```python
from build123d import *

# Parameters (mm, degrees)
SKETCH_1_W          = 3
SKETCH_1_H          = 90
EXTRUDE_1_DEPTH     = 80
SKETCH_2_R          = 2.6
CUT_EXTRUDE_1_DEPTH = 118.276484819
SKETCH_3_W          = 49.268401117
SKETCH_3_H          = 61
CUT_EXTRUDE_2_DEPTH = 118.276484819
SKETCH_4_R          = 2.55
CUT_EXTRUDE_3_DEPTH = 121.608375453
CUT_EXTRUDE_4_DEPTH = 121.608375453
FILLET_2_R          = 5
SKETCH_6_W          = 50
SKETCH_6_H          = 43.1
CUT_EXTRUDE_6_DEPTH = 121.608375453
FILLET_3_R          = 5


with BuildPart() as part:
    # 草图1 → 凸台-拉伸1 (new body)
    with BuildSketch(Plane.XY):
        Polygon((-1.18201613, 42.576507787), (-31.965089897, 81.977045467), (-29.601057636, 83.824029893), (1.18201613, 44.423492213), align=None)
        Rectangle(SKETCH_1_W, SKETCH_1_H)
    extrude(amount=EXTRUDE_1_DEPTH)

    # 草图2 → 切除-拉伸1 (cut, through all)
    with BuildSketch(Plane(origin=(22.285948177, 17.411690984, 0), x_dir=(0.6156614753256597, -0.788010753606721, 0), z_dir=(0.788010753606721, 0.6156614753256597, 0))):
        with Locations(Location((-80.278467782, -4, 0), (0, 0, 180))):
            Circle(SKETCH_2_R)
        with Locations(Location((-80.278467782, -76, 0), (0, 0, 180))):
            Circle(SKETCH_2_R)
        with Locations(Location((-40.278467782, -4, 0), (0, 0, 180))):
            Circle(SKETCH_2_R)
        with Locations(Location((-40.278467782, -76, 0), (0, 0, 180))):
            Circle(SKETCH_2_R)
    extrude(amount=-CUT_EXTRUDE_1_DEPTH, mode=Mode.SUBTRACT)

    # 草图3 → 切除-拉伸2 (cut, through all)
    with BuildSketch(Plane(origin=(22.285948177, 17.411690984, 0), x_dir=(0.6156614753256597, -0.788010753606721, 0), z_dir=(0.788010753606721, 0.6156614753256597, 0))):
        with Locations((-59.644267224, -40)):
            Rectangle(SKETCH_3_W, SKETCH_3_H)
    extrude(amount=-CUT_EXTRUDE_2_DEPTH, mode=Mode.SUBTRACT)

    # 草图4 → 切除-拉伸3 (cut, through all)
    with BuildSketch(Plane(origin=(1.5, 0, 0), x_dir=(0, 0, -1), z_dir=(1, 0, 0))):
        with Locations(Location((-65, -28.3, 0), (0, 0, 90))):
            Circle(SKETCH_4_R)
        with Locations(Location((-65, -41, 0), (0, 0, 90))):
            Circle(SKETCH_4_R)
        with Locations(Location((-52.3, -28.3, 0), (0, 0, 90))):
            Circle(SKETCH_4_R)
        with Locations(Location((-52.3, -41, 0), (0, 0, 90))):
            Circle(SKETCH_4_R)
        with Locations(Location((-39.6, -28.3, 0), (0, 0, 90))):
            Circle(SKETCH_4_R)
        with Locations(Location((-39.6, -41, 0), (0, 0, 90))):
            Circle(SKETCH_4_R)
        with Locations(Location((-26.9, -28.3, 0), (0, 0, 90))):
            Circle(SKETCH_4_R)
        with Locations(Location((-26.9, -41, 0), (0, 0, 90))):
            Circle(SKETCH_4_R)
    extrude(amount=-CUT_EXTRUDE_3_DEPTH, mode=Mode.SUBTRACT)

    # 草图5 → 切除-拉伸4 (cut, through all)
    with BuildSketch(Plane(origin=(1.5, 0, 0), x_dir=(0, 0, -1), z_dir=(1, 0, 0))):
        with BuildLine():
            Line((-80, 6.141923624), (-80, -45))
            Line((-80, -45), (-71.424177932, -45))
            ThreePointArc((-71.424177932, -45), (-70.206204317, -18.505774381), (-80, 6.141923624))
        make_face()
        with BuildLine():
            Line((0, -45), (-8.575822068, -45))
            ThreePointArc((-8.575822068, -45), (-9.793795683, -18.505774381), (0, 6.141923624))
            Line((0, 6.141923624), (0, -45))
        make_face()
    extrude(amount=-CUT_EXTRUDE_4_DEPTH, mode=Mode.SUBTRACT)

    # 圆角2
    # the kernel refuses this fillet: 5 mm, written as the material it adds along each edge
    with BuildSketch(Plane(origin=(-1.5, 42.98350858, 80), x_dir=(-0.61566147532566, 0.7880107536067206, 0), z_dir=(0, 0, -1))) as fillet_2_piece_1_section:
        with BuildLine():
            CenterArc((FILLET_2_R * 0.34432761329, -FILLET_2_R), FILLET_2_R, 90, 38)
            Line((-FILLET_2_R * 0.271333862036, -FILLET_2_R * 0.211989246393), (0, 0))
            Line((0, 0), (FILLET_2_R * 0.34432761329, 0))
        make_face()
    fillet_2_piece_1 = extrude(amount=84.304095166, mode=Mode.PRIVATE)
    fillet_2_piece_1 = split(fillet_2_piece_1, bisect_by=Plane(origin=(-1.5, 42.98350858, 70.5), z_dir=(0, 0, 1)), keep=Keep.TOP, mode=Mode.PRIVATE)
    add(fillet_2_piece_1)
    with BuildSketch(Plane(origin=(-1.5, 42.98350858, 84.304095166), x_dir=(-0.61566147532566, 0.7880107536067206, 0), z_dir=(0, 0, -1))) as fillet_2_piece_2_section:
        with BuildLine():
            CenterArc((FILLET_2_R * 0.34432761329, -FILLET_2_R), FILLET_2_R, 90, 38)
            Line((-FILLET_2_R * 0.271333862036, -FILLET_2_R * 0.211989246393), (0, 0))
            Line((0, 0), (FILLET_2_R * 0.34432761329, 0))
        make_face()
    fillet_2_piece_2 = extrude(amount=84.304095166, mode=Mode.PRIVATE)
    fillet_2_piece_2 = split(fillet_2_piece_2, bisect_by=Plane(origin=(-1.632433378, 43.153015574, 84.304095166), z_dir=(0.6156614753256597, -0.7880107536067209, 0)), keep=Keep.TOP, mode=Mode.PRIVATE)
    fillet_2_piece_2 = split(fillet_2_piece_2, bisect_by=Plane(origin=(-1.5, 42.98350858, 70.5), z_dir=(0, 0, -1)), keep=Keep.TOP, mode=Mode.PRIVATE)
    add(fillet_2_piece_2)
    with BuildSketch(Plane(origin=(-1.5, 42.98350858, 84.304095166), x_dir=(-0.61566147532566, 0.7880107536067206, 0), z_dir=(0, 0, -1))) as fillet_2_piece_3_section:
        with BuildLine():
            CenterArc((FILLET_2_R * 0.34432761329, -FILLET_2_R), FILLET_2_R, 90, 38)
            Line((-FILLET_2_R * 0.271333862036, -FILLET_2_R * 0.211989246393), (0, 0))
            Line((0, 0), (FILLET_2_R * 0.34432761329, 0))
        make_face()
    fillet_2_piece_3 = extrude(amount=84.304095166, mode=Mode.PRIVATE)
    fillet_2_piece_3 = split(fillet_2_piece_3, bisect_by=Plane(origin=(-1.5, 42.98350858, 9.5), z_dir=(0, 0, -1)), keep=Keep.TOP, mode=Mode.PRIVATE)
    add(fillet_2_piece_3)
    # the kernel refuses this fillet: 5 mm, written as the material it takes off along each edge
    with BuildSketch(Plane(origin=(1.5, 45, -6.658439614), x_dir=(0, -1, 0), z_dir=(0, 0, 1))) as fillet_2_2_piece_1:
        with BuildLine():
            CenterArc((2.663375846, -5), FILLET_2_R, 90, 32.186384057)
            Line((0, -0.768401117), (0, 0))
            Line((0, 0), (2.663375846, 0))
        make_face()
    extrude(amount=93.316879228, mode=Mode.SUBTRACT)

    # 草图6 → 切除-拉伸6 (cut, through all)
    with BuildSketch(Plane(origin=(1.5, 0, 0), x_dir=(0, 0, -1), z_dir=(1, 0, 0))):
        with Locations((-39.698542008, 15.9)):
            Rectangle(SKETCH_6_W, SKETCH_6_H)
    extrude(amount=-CUT_EXTRUDE_6_DEPTH, mode=Mode.SUBTRACT)

    # 圆角3
    # the kernel refuses this fillet: 5 mm, written as the material it adds along each edge
    with BuildSketch(Plane(origin=(1.5, -5.65, 14.698542008), x_dir=(0, 1, 0), z_dir=(-1, 0, 0)), Plane(origin=(1.5, -5.65, 64.698542008), x_dir=(0, 0, -1), z_dir=(-1, 0, 0)), Plane(origin=(1.5, 37.45, 64.698542008), x_dir=(0, -1, 0), z_dir=(-1, 0, 0))) as fillet_3_piece_1:
        with BuildLine():
            CenterArc((FILLET_3_R, -FILLET_3_R), FILLET_3_R, 90, 90)
            Line((0, -FILLET_3_R), (0, 0))
            Line((0, 0), (FILLET_3_R, 0))
        make_face()
    extrude(amount=3)
    with BuildSketch(Plane(origin=(1.5, 37.45, 14.698542008), x_dir=(0, -1, 0), z_dir=(-1, 0, 0))) as fillet_3_piece_2:
        with BuildLine():
            CenterArc((FILLET_3_R, FILLET_3_R), FILLET_3_R, 180, 90)
            Line((0, FILLET_3_R), (0, 0))
            Line((0, 0), (FILLET_3_R, 0))
        make_face()
    extrude(amount=3)
    # the kernel refuses this fillet: 5 mm, written as the material it takes off along each edge
    with BuildSketch(Plane(origin=(-41.815224317, 74.281277026, 0), x_dir=(0.6156614753256596, -0.7880107536067208, 0), z_dir=(0.7880107536067208, 0.6156614753256597, 0)), Plane(origin=(-19.750923216, 91.519798335, 9.5), x_dir=(0.6156614753256597, -0.7880107536067208, 1.0658141036401496e-15), z_dir=(-0.7880107536067209, -0.6156614753256597, 0))) as fillet_3_2_piece_1:
        with BuildLine():
            CenterArc((FILLET_3_R, -FILLET_3_R), FILLET_3_R, 90, 90)
            Line((0, -FILLET_3_R), (0, 0))
            Line((0, 0), (FILLET_3_R, 0))
        make_face()
    extrude(amount=28, mode=Mode.SUBTRACT)
    with BuildSketch(Plane(origin=(-41.815224317, 74.281277026, 80), x_dir=(0.6156614753256597, -0.7880107536067208, 0), z_dir=(0.7880107536067208, 0.6156614753256597, 0)), Plane(origin=(-19.750923216, 91.519798335, 70.5), x_dir=(0.6156614753256597, -0.7880107536067208, 0), z_dir=(-0.7880107536067209, -0.6156614753256597, 0))) as fillet_3_2_piece_2:
        with BuildLine():
            CenterArc((FILLET_3_R, FILLET_3_R), FILLET_3_R, 180, 90)
            Line((0, FILLET_3_R), (0, 0))
            Line((0, 0), (FILLET_3_R, 0))
        make_face()
    extrude(amount=28, mode=Mode.SUBTRACT)
    with BuildSketch(Plane(origin=(5.221396316, 6.141923624, 0), x_dir=(0, 1, 0), z_dir=(-1, 0, 0))) as fillet_3_2_piece_3:
        with BuildLine():
            CenterArc((1.488558526, -5), FILLET_3_R, 90, 32.518664638)
            ThreePointArc((-1.199313086, -0.783918147), (-0.597427923, -0.395368629), (0, 0))
            Line((0, 0), (1.488558526, 0))
        make_face()
    extrude(amount=10.442792632, mode=Mode.SUBTRACT)
    with BuildSketch(Plane(origin=(5.221396316, 6.141923624, 80), x_dir=(0, 1, 0), z_dir=(-1, 0, 0))) as fillet_3_2_piece_4:
        with BuildLine():
            CenterArc((1.488558526, 5), FILLET_3_R, 237.481335362, 32.518664638)
            ThreePointArc((-1.199313086, 0.783918147), (-0.597427923, 0.395368629), (0, 0))
            Line((0, 0), (1.488558526, 0))
        make_face()
    extrude(amount=10.442792632, mode=Mode.SUBTRACT)
    with BuildSketch(Plane(origin=(16.943632487, -45, 71.424177932), x_dir=(0, 0, -1), z_dir=(-1, 0, 0))) as fillet_3_2_piece_5:
        with BuildLine():
            CenterArc((6.177452995, -5), FILLET_3_R, 90, 99.373749783)
            ThreePointArc((1.244218563, -5.814369722), (0.69074329, -2.892497851), (0, 0))
            Line((0, 0), (6.177452995, 0))
        make_face()
    extrude(amount=33.887264974, mode=Mode.SUBTRACT)
    with BuildSketch(Plane(origin=(16.943632487, -45, 8.575822068), x_dir=(0, 0.9778615645016191, 0.20925286299223153), z_dir=(-1, 0, 0))) as fillet_3_2_piece_6:
        with BuildLine():
            CenterArc((6.181957548, -4.994429535), FILLET_3_R, 92.704821928, 99.373749783)
            Line((1.292649725, -6.04069385), (0, 0))
            ThreePointArc((0, 0), (2.973002485, -0.070187858), (5.946004969, 0))
        make_face()
    extrude(amount=33.887264974, mode=Mode.SUBTRACT)


solid = part.part
```
Build history of the part. All positions in model axes, mm. A direction names the side the tool comes from. Coordinates: 2 decimals unless noted, no trailing zeros. Write each loop counter-clockwise with the first axis right and the second up, starting at its lowest first coordinate (ties: lowest second). Pieces come first, ordered by that corner, then holes.
1. Band-saw the part on D-D, the plane z = 18. Give the cut face in (x, y), and give its area (3 significant figures).
Answer block:
outline: (-1.82, 43.01) arc R5 cw to (-1.5, 41.26) - (-1.5, 37.15) - (1.5, 37.15) - (1.5, 42.34) arc R5 ccw to (0.73, 45) - close; (-1.5, -45) - (1.5, -45) - (1.5, -5.35) - (-1.5, -5.35) - close
area: 140 mm2
2. 3-axis set-ups, long thin cutter, end or side, ignore diameter. For faces 5 (the flat face through (-0.52, 44.02, 39.57)), 6 (the cylindrical face through (-29.82, 81.63, 1.34)), 7 (the cylindrical face through (0.02, 35.95, 63.27)): which of +Z, -Z, +X, -X, +Y, -Y reach the whole face in a straight line?
Answer block:
face 5: -X, +Y
face 6: -Z, -X, +Y
face 7: +X, -X
3. Band-saw the part on A-A, the plane y = 22. Give the cut face in (x, z).
Answer block:
outline: (-1.5, 0) - (1.5, 0) - (1.5, 14.7) - (-1.5, 14.7) - close; (-1.5, 64.7) - (1.5, 64.7) - (1.5, 80) - (-1.5, 80) - close
4. Drop flat-ended pins along their axis: pin 1 (5 mm diameter, centred on x = -22, z = 66.5, fed in from -Y); pin 2 (2 mm diameter, centred on y = -24.5, z = 64.5, fed in from -X); pin 3 (0.9 mm diameter, centred on x = -0.5, z = 47, fed in from +Y). Give the stop position or say it passes through.
Answer block:
pin 1: passes through
pin 2: stops at x = -1.5
pin 3: stops at y = 44.39
5. Band-saw the part on B-B, the plane z = 52.3. Give the cut face in (x, y), and give its area (3 significant figures).
Answer block:
outline: (-1.82, 43.01) arc R5 cw to (-1.5, 41.26) - (-1.5, 37.45) - (1.5, 37.45) - (1.5, 42.34) arc R5 ccw to (0.73, 45) - close; (-1.5, -45) - (1.5, -45) - (1.5, -43.55) - (-1.5, -43.55) - close; (-1.5, -38.45) - (1.5, -38.45) - (1.5, -30.85) - (-1.5, -30.85) - close; (-1.5, -25.75) - (1.5, -25.75) - (1.5, -5.65) - (-1.5, -5.65) - close
area: 108 mm2
6. Band-saw the part on C-C, the plane x = -14. Give the cut face in (y, z).
Answer block:
outline: (58.98, 0) - (63.86, 0) - (63.86, 9.5) - (58.98, 9.5) - close; (58.98, 70.5) - (63.86, 70.5) - (63.86, 80) - (58.98, 80) - close
7. Drill centre lines: probe 1 along Z at (x, y) = (0, -28); probe 2 along Y at (x, z) = (-0.5, 41.5); probe 3 along Z at (x, y) = (0, -41). Where is each one in solid material? Low to high.
Answer block:
probe 1: z = 10.65 to 24.37, 29.43 to 37.07, 42.13 to 49.77, 54.83 to 62.47, 67.53 to 69.35
probe 2: y = -45 to -42.7, -39.3 to -30, -26.6 to -5.65, 37.45 to 44.04
probe 3: z = 9.85 to 24.35, 29.45 to 37.05, 42.15 to 49.75, 54.85 to 62.45, 67.55 to 70.15
8. Pull direction Y, two halves, no side cores. Call faces 1 (the cylindrical face through (0.021, 6.25, 0.194)), 2 (the flat face through (0, -5.65, 40)), 3 (the flat face through (-4, 47, 0)), 4 (the flat face through (-14.645, 64.681, 75.184)): released by +Y, released by -Y, zero draft, split by the parting line, or undercut.
Answer block:
face 1: released by -Y
face 2: undercut
face 3: zero draft
face 4: released by +Y
